```python
from build123d import *

# Parameters (mm, degrees)
SKETCH034_W          = 20.3
SKETCH034_H          = 20.3
PAD005_DEPTH         = 10
SKETCH035_W          = 3.2
SKETCH035_H          = 10
POCKET026_DEPTH      = 7
FILLET002_R          = 1
SKETCH036_R          = 1.6
POCKET027_DEPTH      = 12.501
POCKET027_DEPTH_BACK = 12.501


with BuildPart() as part:
    # Sketch034 → Pad005 (new body)
    with BuildSketch(Plane.XY):
        Polygon((-12.5, 12.5), (-4.5, 12.5), (-4.5, 22.5), (4.5, 22.5), (4.5, 12.5), (12.5, 12.5), (12.5, -12.5), (-12.5, -12.5), align=None)
        Rectangle(SKETCH034_W, SKETCH034_H, mode=Mode.SUBTRACT)
    extrude(amount=PAD005_DEPTH)

    # Sketch035 → Pocket026 (cut)
    with BuildSketch(Plane.XY.offset(3)):
        with Locations((0, 17.5)):
            Rectangle(SKETCH035_W, SKETCH035_H)
    extrude(amount=POCKET026_DEPTH, mode=Mode.SUBTRACT)

    # Fillet002
    fillet002_edges = [part.edges().sort_by_distance(p)[0] for p in [
        (1.6, 22.5, 6.5),
        (1.6, 17.5, 10),
        (-1.6, 22.5, 6.5),
        (-1.6, 17.5, 10),
    ]]
    fillet(fillet002_edges, radius=FILLET002_R)

    # Sketch036 → Pocket027 (cut, two sides)
    with BuildSketch(Plane.YZ) as pocket027_sk:
        with Locations((0, 5)):
            Circle(SKETCH036_R)
    extrude(amount=-POCKET027_DEPTH, mode=Mode.SUBTRACT)
    extrude(pocket027_sk.sketch, amount=POCKET027_DEPTH_BACK, mode=Mode.SUBTRACT)


solid = part.part
```
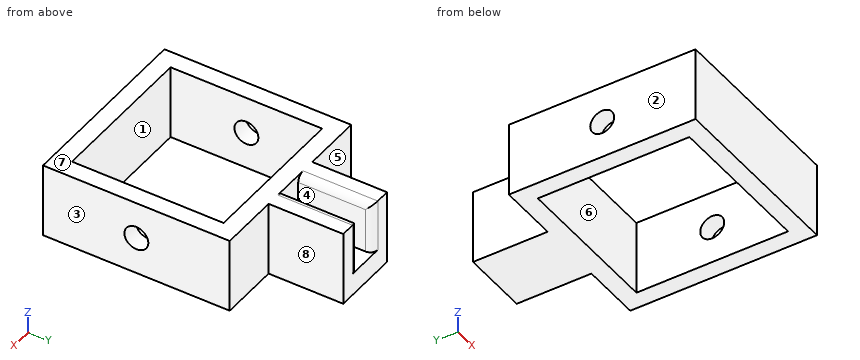
Source: CAD feature listing. Evaluate the final solid. Frame: model axes, mm. Face numbers are marked on the shaded views. A direction names the side the tool comes from. Give positions to 0.01 mm unless a question says otherwise; leave off trailing zeros. Order: outer loops, then holes, each group sorted by start corner. A loop starts at its lowest first (then second) coordinate and runs counter-clockwise, first axis right, second up. Notation, with made-up numbers: (8.5, 51) -> (30.5, 51) arc R15 ccw to (30.5, 55) -> close; hole circle Ø8 at (5, -18). An arc over 180 degrees is marked (long way). Use a Markdown table: item, result.
Q1. Pull-direction query (X, two-part tool) for the marked faces 1, 2 and 3; classes: +X half, -X half, draft (parallel to the pull), parting line (faces both ways), or undercut.
A:
| item | result |
|---|---|
| face 1 | undercut |
| face 2 | -X half |
| face 3 | +X half |
Q2. Material intervals for line 1 (X direction, y = 3, z = 1); line 2 (Z direction, x = 11.4, y = 0), sorted ascending. Write a range as [from, to].
A:
| item | result |
|---|---|
| line 1 | [-12.5, -10.15], [10.15, 12.5] |
| line 2 | [0, 3.4], [6.6, 10] |
Q3. First-contact query: P1, Ø12, axis at x = -1.5, y = 2.5, coming from the +Z side; P2, Ø5, axis at y = 17, z = 6, coming from the +X side; P3, Ø5, axis at y = 19, z = 6.5, coming from the -X side; P4, Ø2.5, axis at x = 8, z = 4, coming from the +Y side. Flat tips, straight axial feed; report the tip coordinate or a pass-through.
A:
| item | result |
|---|---|
| P1 | through |
| P2 | x = 4.5 |
| P3 | x = -4.5 |
| P4 | y = 12.5 |
Q4. Access query for the marked faces 4, 5, 6, 7 and 8. Directions: +Z, -Z, +X, -X, +Y, -Y. A direction counts if a zero-diameter tool reaches every point of the face in a straight line with its end or side. Return the directions, or none.
A:
| item | result |
|---|---|
| face 4 | +Z, +Y |
| face 5 | +Z, -Z, -X, +Y |
| face 6 | +Z, -Z |
| face 7 | +Z, +X, -X, +Y, -Y |
| face 8 | +Z, -Z, +X, +Y |
Q5. Section C-C (z = 5). Return the cut outline in (x, y).
A:
| item | result |
|---|---|
| outline | (-12.5, -12.5) -> (12.5, -12.5) -> (12.5, -1.6) -> (10.15, -1.6) -> (10.15, -10.15) -> (-10.15, -10.15) -> (-10.15, -1.6) -> (-12.5, -1.6) -> close; (-12.5, 1.6) -> (-10.15, 1.6) -> (-10.15, 10.15) -> (10.15, 10.15) -> (10.15, 1.6) -> (12.5, 1.6) -> (12.5, 12.5) -> (4.5, 12.5) -> (4.5, 22.5) -> (2.6, 22.5) arc R1 ccw to (1.6, 21.5) -> (1.6, 12.5) -> (-1.6, 12.5) -> (-1.6, 21.5) arc R1 ccw to (-2.6, 22.5) -> (-4.5, 22.5) -> (-4.5, 12.5) -> (-12.5, 12.5) -> close |
Q6. Section A-A (y = 0). Return the cut outline in (x, z), and give its area (3 significant figures).
A:
| item | result |
|---|---|
| outline | (-12.5, 0) -> (-10.15, 0) -> (-10.15, 3.4) -> (-12.5, 3.4) -> close; (-12.5, 6.6) -> (-10.15, 6.6) -> (-10.15, 10) -> (-12.5, 10) -> close; (10.15, 0) -> (12.5, 0) -> (12.5, 3.4) -> (10.15, 3.4) -> close; (10.15, 6.6) -> (12.5, 6.6) -> (12.5, 10) -> (10.15, 10) -> close |
| area | 32.0 mm^2 |
Q7. Section B-B (x = -5.75). Return the cut outline in (y, z), and give its area (3 significant figures).
A:
| item | result |
|---|---|
| outline | (-12.5, 0) -> (-10.15, 0) -> (-10.15, 10) -> (-12.5, 10) -> close; (10.15, 0) -> (12.5, 0) -> (12.5, 10) -> (10.15, 10) -> close |
| area | 47.0 mm^2 |
